Job drawing, mm, ordinate dimensions from the low corner. One solid piece. Give positions to 0.01 mm unless a question says otherwise; leave off trailing zeros. Loops run counter-clockwise (first coordinate to the right, second up) from the corner with the lowest first, then second, coordinate; pieces in that order, holes last. Notation, with made-up numbers: (-35.5, 86) -> (11.5, 86) arc R23 cw to (11.5, 103) -> close; hole circle Ø9 at (80.5, 1.5). An arc over 180 degrees is marked (long way). Use one line per item in the form item = value.
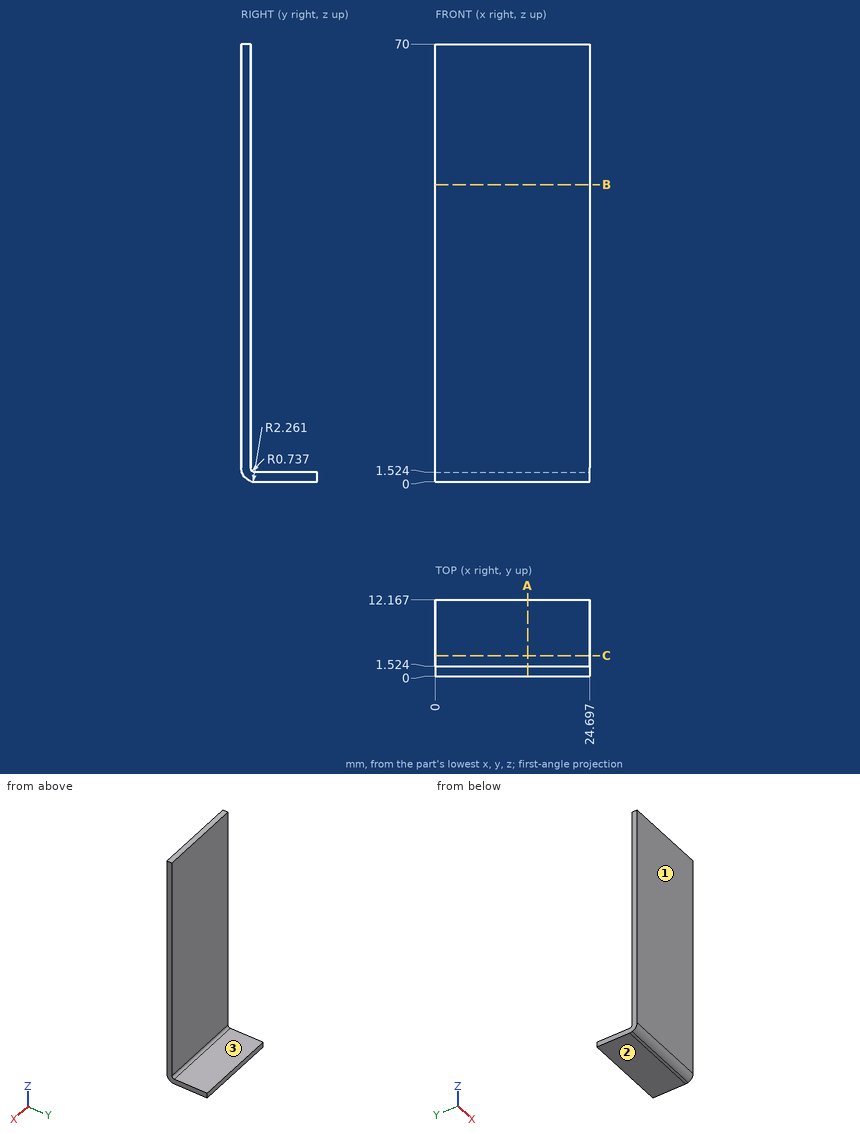
1. Drop flat-ended pins along their axis: P1, Ø1.5, axis at x = 22, z = 15, coming from the +Y side; P2, Ø5, axis at x = 7, y = 5, coming from the +Z side; P3, Ø3, axis at x = 21.5, y = 5, coming from the -Z side. Give the stop position or say it passes through.
Result sheet:
P1 = 1.52
P2 = 1.52
P3 = 0
2. Drill centre lines: line 1 (Y direction, x = 2, z = 24); line 2 (Z direction, x = 18.5, y = 0.75). Where is each one in solid material? Low to high.
Result sheet:
line_1 = 0 to 1.52
line_2 = 0.58 to 70
3. Cut at A-A, the plane x = 14.75. Write the cut outline in (y, z), then the cut area to 3 significant figures.
Result sheet:
outline = (0, 2.26) arc R2.26 ccw to (2.26, 0) -> (12.17, 0) -> (12.17, 1.52) -> (2.26, 1.52) arc R0.74 cw to (1.52, 2.26) -> (1.52, 70) -> (0, 70) -> close
area = 122 mm^2
4. Cut at B-B, the plane z = 47.5. Write the cut outline in (x, y).
Result sheet:
outline = (0, 0) -> (24.7, 0) -> (24.7, 1.52) -> (0, 1.52) -> close
5. Mould opens along Z. For the marked faces 1, 2 and 3 say: pulls with the +Z half, pulls with the -Z half, needs draft (parallel to the pull), parting line crosses it, or undercut.
Result sheet:
face_1 = needs draft
face_2 = pulls with the -Z half
face_3 = pulls with the +Z half
